```python
from build123d import *

# Parameters (mm, degrees)
SKETCH_1_W          = 7.8
SKETCH_1_H          = 5.08
EXTRUDE_1_DEPTH     = 12
SKETCH_2_R          = 0.5
CUT_EXTRUDE_1_DEPTH = 12
SKETCH_3_R          = 0.875
CUT_EXTRUDE_2_DEPTH = 0.1
CUT_EXTRUDE_START   = -10
SKETCH_4_W          = 1.5
SKETCH_4_H          = 2
CUT_EXTRUDE_3_DEPTH = 10


with BuildPart() as part:
    # 草图1 → 拉伸1 (new body)
    with BuildSketch(Plane(origin=(0, 0, 0), x_dir=(1, 0, 0), z_dir=(0, 1, 0))):
        Rectangle(SKETCH_1_W, SKETCH_1_H)
    extrude(amount=EXTRUDE_1_DEPTH)

    # 草图2 → 切除-拉伸1 (cut)
    with BuildSketch(Plane(origin=(0, 12, 0), x_dir=(1, 0, 0), z_dir=(0, 1, 0))):
        with Locations(Location((0, 0, 0), (0, 0, 270))):
            Circle(SKETCH_2_R)
    extrude(amount=-CUT_EXTRUDE_1_DEPTH, mode=Mode.SUBTRACT)

    # 草图3 → 切除-拉伸2 (cut)
    with BuildSketch(Plane(origin=(0, 12, 0), x_dir=(1, 0, 0), z_dir=(0, 1, 0))):
        with Locations(Location((0, 0, 0), (0, 0, 270))):
            Circle(SKETCH_3_R)
    extrude(amount=-CUT_EXTRUDE_2_DEPTH, mode=Mode.SUBTRACT)

    # 草图4 → 切除-拉伸3 (cut)
    with BuildSketch(Plane.XZ.offset(CUT_EXTRUDE_START)):
        with Locations((-2.65, 0)):
            Rectangle(SKETCH_4_W, SKETCH_4_H)
        with Locations((2.65, 0)):
            Rectangle(SKETCH_4_W, SKETCH_4_H)
    extrude(amount=CUT_EXTRUDE_3_DEPTH, mode=Mode.SUBTRACT)


solid = part.part
```
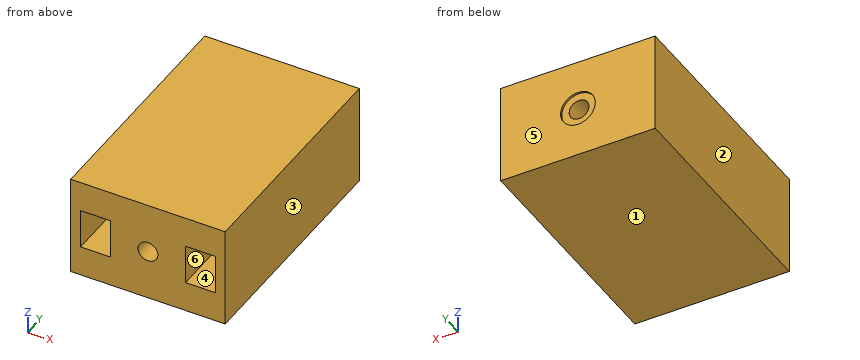
Can you work these out from the model? Positions are in its coordinate system, mm. Face numbers are marked on the shaded views. A direction names the side the tool comes from. Round coordinates to 2 decimals unless told otherwise and drop trailing zeros. Order: outer loops, then holes, each group sorted by start corner. A loop starts at its lowest first (then second) coordinate and runs counter-clockwise, first axis right, second up.
(1) If we section it at A-A (x = 0): Please give me the cut outline in (y, z) (3 decimals), plus the area to 3 significant figures.
Results are:
outline: (0, -2.54) - (12, -2.54) - (12, -0.875) - (11.9, -0.875) - (11.9, -0.5) - (0, -0.5) - close; (0, 0.5) - (11.9, 0.5) - (11.9, 0.875) - (12, 0.875) - (12, 2.54) - (0, 2.54) - close
area: 48.9 mm2
(2) If we section it at D-D (x = 2.5): Please give me the cut outline in (y, z), plus the area to 3 significant figures.
Results are:
outline: (0, -2.54) - (12, -2.54) - (12, 2.54) - (0, 2.54) - (0, 1) - (10, 1) - (10, -1) - (0, -1) - close
area: 41.0 mm2
(3) I'm going to push flat-ended pins straight in: pin 1 (1.1 mm diameter, centred on x = 0, z = 0, fed in from +Y); pin 2 (0.8 mm diameter, centred on x = -2.5, z = 0.5, fed in from -Y). Where does each tip first touch, or does it pass through?
Results are:
pin 1: stops at y = 11.9
pin 2: stops at y = 10
(4) We'd pull the mould along X, two halves only. Please class the marked faces 1, 2, 3 and 4: +X half, -X half, draft (parallel to the pull), parting line (faces both ways), or undercut.
Results are:
face 1: draft
face 2: -X half
face 3: +X half
face 4: undercut
(5) If we section it at C-C (z = 0): Please give me the cut outline in (x, y) (3 decimals), plus the area to 3 significant figures.
Results are:
outline: (-3.9, 0) - (-3.4, 0) - (-3.4, 10) - (-1.9, 10) - (-1.9, 0) - (-0.5, 0) - (-0.5, 11.9) - (-0.875, 11.9) - (-0.875, 12) - (-3.9, 12) - close; (0.5, 0) - (1.9, 0) - (1.9, 10) - (3.4, 10) - (3.4, 0) - (3.9, 0) - (3.9, 12) - (0.875, 12) - (0.875, 11.9) - (0.5, 11.9) - close
area: 51.5 mm2
(6) If I drill on L1, parallel to X at y = 2.5, z = 0.7; L2, parallel to X at y = 4.5, z = 0; L3, parallel to Y at x = -2, z = 0.3, over which ranges is the centre line in solid material (lowest first)?
Results are:
L1: x = -3.9 to -3.4, -1.9 to 1.9, 3.4 to 3.9
L2: x = -3.9 to -3.4, -1.9 to -0.5, 0.5 to 1.9, 3.4 to 3.9
L3: y = 10 to 12
(7) If we section it at B-B (y = 4): Please give me the cut outline in (x, z).
Results are:
outline: (-3.9, -2.54) - (3.9, -2.54) - (3.9, 2.54) - (-3.9, 2.54) - close; hole (-3.4, -1) - (-1.9, -1) - (-1.9, 1) - (-3.4, 1) - close; hole circle Ø1 at (0, 0); hole (1.9, -1) - (3.4, -1) - (3.4, 1) - (1.9, 1) - close
(8) On a 3-axis mill with a long thin cutter (end or side, diameter ignored), from which of +Z, -Z, +X, -X, +Y, -Y can I reach the whole of each face in a straight line? I mean the marked faces 5 and 6. Say none if no direction works.
Results are:
face 5: +Z, -Z, +X, -X, +Y
face 6: -Y
